Can you work these out from the model? Positions are in its coordinate system, mm. A direction names the side the tool comes from. Give positions to 0.01 mm unless a question says otherwise; leave off trailing zeros. Order: outer loops, then holes, each group sorted by start corner. A loop starts at its lowest first (then second) coordinate and runs counter-clockwise, first axis right, second up.
Item 1: I want a section at C-C, the plane z = 8. Write out the boundary of the cut face in (x, y).
Item 2: If we mould it in two halves opening along Z, with no side actions, what happens to faces 4 (the flat face through (0, 13, 15)), 5 (the flat face through (-17, 9, 0)), 6 (the flat face through (0, 9, 2))? For each: +Z half, -Z half, draft (parallel to the pull), parting line (faces both ways), or undercut.
Item 3: Which directions (+Z, -Z, +X, -X, +Y, -Y) give clear straight access to the entire face, cutting with the end or side of a thin tool? Please do faces 1 (the flat face through (0, 16.95, -4)), 2 (the cylindrical face through (1.352, -0.126, 4.292)), 3 (the flat face through (16, 9, 0)).
Item 4: I want a section at D-D, the plane x = -15.5. Write out the boundary of the cut face in (y, z).
Item 5: I'm going to push flat-ended pins straight in: pin 1 Ø4.5 at (x, z) = (0, 0) entering from +Y; pin 2 Ø4.5 at (x, z) = (1, 1) entering from -Y; pin 3 Ø2 at (y, z) = (1, 0.5) entering from -X. Where does each tip first touch, or does it pass through?
Item 6: If I drill on line 1 along X through (y, z) = (1.75, 0); line 2 along Z through (x, y) = (0, 12.75); line 3 along Y through (x, z) = (16.5, -1), over which ranges is the centre line in solid material (lowest first)?
Item 7: I want a section at B-B, the plane y = 3.75. Write out the boundary of the cut face in (x, z).
Item 8: I want a section at A-A, the plane z = 0. Write out the boundary of the cut face in (x, y).
```python
from build123d import *

# Parameters (mm, degrees)
SKETCH1_R                                           = 15
SKETCH1_R_2                                         = 4.5
BOSS_EXTRUDE1_DEPTH                                 = 9
SKETCH2_W                                           = 39.8
SKETCH2_H                                           = 30
SKETCH2_R                                           = 1.5
BOSS_EXTRUDE2_DEPTH                                 = 7.95
CSK_FOR_M3_COUNTERSUNK_FLAT_HEAD_SCREW1_D           = 3.4
CSK_FOR_M3_COUNTERSUNK_FLAT_HEAD_SCREW1_CSINK_D     = 6.3
CSK_FOR_M3_COUNTERSUNK_FLAT_HEAD_SCREW1_CSINK_ANGLE = 90
M5_TAPPED_HOLE1_REACH                               = 45.286
M5_TAPPED_HOLE1_BORE_R                              = 2.1
M5_TAPPED_HOLE2_REACH                               = 45.286
M5_TAPPED_HOLE2_BORE_R                              = 2.1


with BuildPart() as part:
    # Sketch1 → Boss-Extrude1 (new, symmetric)
    with BuildSketch(Plane(origin=(0, 0, 0), x_dir=(1, 0, 0), z_dir=(0, 1, 0))):
        with Locations(Location((0, 0, 0), (0, 0, 270))):
            Circle(SKETCH1_R)
        with Locations(Location((0, 0, 0), (0, 0, 270))):
            Circle(SKETCH1_R_2, mode=Mode.SUBTRACT)
    extrude(amount=BOSS_EXTRUDE1_DEPTH, both=True)

    # Sketch2 → Boss-Extrude2 (add)
    with BuildSketch(Plane(origin=(0, 9, 0), x_dir=(1, 0, 0), z_dir=(0, 1, 0))):
        Rectangle(SKETCH2_W, SKETCH2_H)
        with Locations(Location((0, 0, 0), (0, 0, 270))):
            Circle(SKETCH2_R, mode=Mode.SUBTRACT)
    extrude(amount=BOSS_EXTRUDE2_DEPTH)

    # CSK for M3 Countersunk Flat Head Screw1 (through all)
    with Locations(Plane(origin=(0, 16.95, 0), x_dir=(1, 0, 0), z_dir=(0, 1, 0))):
        with Locations((0, 0)):
            CounterSinkHole(CSK_FOR_M3_COUNTERSUNK_FLAT_HEAD_SCREW1_D / 2, CSK_FOR_M3_COUNTERSUNK_FLAT_HEAD_SCREW1_CSINK_D / 2, counter_sink_angle=CSK_FOR_M3_COUNTERSUNK_FLAT_HEAD_SCREW1_CSINK_ANGLE)

    # M5 Tapped Hole1 bore → M5 Tapped Hole1 (cut, up to next)
    with BuildSketch(Plane(origin=(10.606601718, 0, -10.606601718), x_dir=(-0.7071067811865476, 0, -0.7071067811865476), z_dir=(0.7071067811865476, 0, -0.7071067811865476)), mode=Mode.PRIVATE) as m5_tapped_hole1_sk1:
        with Locations((0, -4)):
            Circle(M5_TAPPED_HOLE1_BORE_R)
    m5_tapped_hole1_tool1 = extrude(m5_tapped_hole1_sk1.sketch, amount=-M5_TAPPED_HOLE1_REACH, mode=Mode.PRIVATE) & part.part
    add(m5_tapped_hole1_tool1.solids().sort_by_distance((10.606602, -4, -10.606602))[0], mode=Mode.SUBTRACT)

    # M5 Tapped Hole2 bore → M5 Tapped Hole2 (cut, up to next)
    with BuildSketch(Plane(origin=(-10.606601718, 0, -10.606601718), x_dir=(-0.7071067811865476, 0, 0.7071067811865476), z_dir=(-0.7071067811865476, 0, -0.7071067811865476)), mode=Mode.PRIVATE) as m5_tapped_hole2_sk1:
        with Locations((0, -4)):
            Circle(M5_TAPPED_HOLE2_BORE_R)
    m5_tapped_hole2_tool1 = extrude(m5_tapped_hole2_sk1.sketch, amount=-M5_TAPPED_HOLE2_REACH, mode=Mode.PRIVATE) & part.part
    add(m5_tapped_hole2_tool1.solids().sort_by_distance((-10.606602, -4, -10.606602))[0], mode=Mode.SUBTRACT)


solid = part.part
```
Results list:
1. outline: (-19.9, 9) - (-12.69, 9) - (-12.69, -9) - (12.69, -9) - (12.69, 9) - (19.9, 9) - (19.9, 16.95) - (-19.9, 16.95) - close
2. face 4: +Z half
2. face 5: draft
2. face 6: undercut
3. face 1: +Z, -Z, +X, -X, +Y
3. face 2: -Y
3. face 3: +X, -Y
4. outline: (9, -15) - (16.95, -15) - (16.95, 15) - (9, 15) - close
5. pin 1: stops at y = 16.05
5. pin 2: stops at y = 9
5. pin 3: stops at x = -15
6. line 1: x = -15 to -4.5, 4.5 to 15
6. line 2: z = -15 to -1.7, 1.7 to 15
6. line 3: y = 9 to 16.95
7. outline: circle Ø30 at (0, 0); hole circle Ø9 at (0, 0)
8. outline: (-19.9, 9) - (-15, 9) - (-15, -9) - (-4.5, -9) - (-4.5, 9) - (-1.7, 9) - (-1.7, 15.5) - (-3.15, 16.95) - (-19.9, 16.95) - close; (1.7, 9) - (4.5, 9) - (4.5, -9) - (15, -9) - (15, 9) - (19.9, 9) - (19.9, 16.95) - (3.15, 16.95) - (1.7, 15.5) - close
